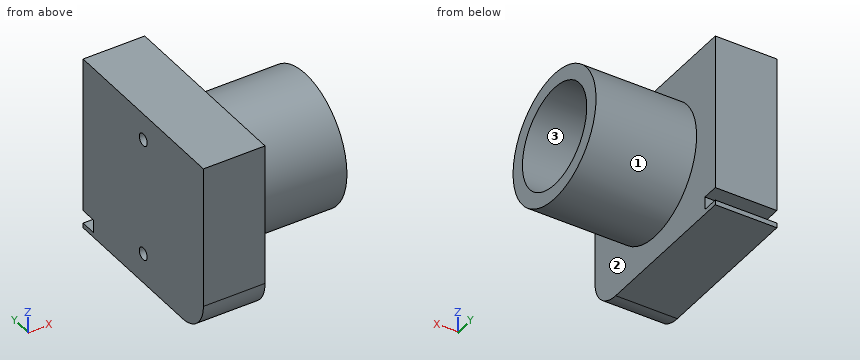
from build123d import *

# Parameters (mm, degrees)
SKETCH1_W           = 19
SKETCH1_H           = 58
BOSS_EXTRUDE1_DEPTH = 54
SKETCH2_3_R         = 20
SKETCH2_3_R_2       = 15.5
BOSS_EXTRUDE2_DEPTH = 50
SKETCH2_R           = 1.9
CUT_EXTRUDE1_DEPTH  = 10
FILLET1_R           = 10
BOSS_EXTRUDE3_DEPTH = 50
SKETCH4_R           = 1.25
CUT_EXTRUDE2_DEPTH  = 55
SKETCH5_W           = 17
SKETCH5_H           = 14
CUT_EXTRUDE3_DEPTH  = 2
SKETCH6_W           = 19
SKETCH6_H           = 4
CUT_EXTRUDE4_DEPTH  = 5
SKETCH7_W           = 17
SKETCH7_H           = 14
CUT_EXTRUDE5_DEPTH  = 53


with BuildPart() as part:
    # Sketch1 → Boss-Extrude1 (new body)
    with BuildSketch(Plane.XY):
        with Locations((9.5, 29)):
            Rectangle(SKETCH1_W, SKETCH1_H)
    extrude(amount=BOSS_EXTRUDE1_DEPTH)

    # Sketch2<3> → Boss-Extrude2 (add)
    with BuildSketch(Plane.ZY):
        with Locations((27.5, 29)):
            Circle(SKETCH2_3_R)
        with Locations((27.5, 29)):
            Circle(SKETCH2_3_R_2, mode=Mode.SUBTRACT)
    extrude(amount=-BOSS_EXTRUDE2_DEPTH)

    # Sketch2 → Cut-Extrude1 (cut)
    with BuildSketch(Plane.ZY):
        with Locations((9.25, 29)):
            Circle(SKETCH2_R)
        with Locations((45.75, 29)):
            Circle(SKETCH2_R)
    extrude(amount=-CUT_EXTRUDE1_DEPTH, mode=Mode.SUBTRACT)

    # Fillet1
    fillet1_edges = [part.edges().sort_by_distance(p)[0] for p in [
        (9.5, 0, 0),
    ]]
    fillet(fillet1_edges, radius=FILLET1_R)

    # Sketch3 → Boss-Extrude3 (add)
    with BuildSketch(Plane(origin=(0, 0, 0), x_dir=(0, 0, -1), z_dir=(1, 0, 0))):
        Polygon((0, 0), (0, 57), (0, 67), (-5, 67), (-5, 0), align=None)
    extrude(amount=-BOSS_EXTRUDE3_DEPTH)

    # Sketch4 → Cut-Extrude2 (cut, through all)
    with BuildSketch(Plane(origin=(0, 0, 0), x_dir=(-1, 0, 0), z_dir=(0, 0, -1))):
        with Locations((14, 57)):
            Circle(SKETCH4_R)
        Polygon((0, 53), (0, 0), (50, 0), (50, 67), (17, 67), (17, 53), align=None)
        with Locations((14, 63.5)):
            Circle(SKETCH4_R)
    extrude(amount=-CUT_EXTRUDE2_DEPTH, mode=Mode.SUBTRACT)

    # Sketch5 → Cut-Extrude3 (cut)
    with BuildSketch(Plane(origin=(0, 0, 0), x_dir=(-1, 0, 0), z_dir=(0, 0, -1))):
        with Locations((8.5, 60)):
            Rectangle(SKETCH5_W, SKETCH5_H)
    extrude(amount=-CUT_EXTRUDE3_DEPTH, mode=Mode.SUBTRACT)

    # Sketch6 → Cut-Extrude4 (cut)
    with BuildSketch(Plane(origin=(0, 58, 0), x_dir=(1, 0, 0), z_dir=(0, 1, 0))):
        with Locations((9.5, -3.5)):
            Rectangle(SKETCH6_W, SKETCH6_H)
    extrude(amount=-CUT_EXTRUDE4_DEPTH, mode=Mode.SUBTRACT)

    # Sketch7 → Cut-Extrude5 (cut, through all)
    with BuildSketch(Plane(origin=(0, 0, 2), x_dir=(-1, 0, 0), z_dir=(0, 0, -1))):
        with Locations((8.5, 60)):
            Rectangle(SKETCH7_W, SKETCH7_H)
    extrude(amount=-CUT_EXTRUDE5_DEPTH, mode=Mode.SUBTRACT)


solid = part.part
Check sheet for the modelled part. Datum: model origin and axes. Units: mm. Face numbers are marked on the shaded views. Give positions to 0.01 mm unless a question says otherwise; leave off trailing zeros. Write each loop counter-clockwise with the first axis right and the second up, starting at its lowest first coordinate (ties: lowest second). Pieces come first, ordered by that corner, then holes. Notation, with made-up numbers: (29, -3) -> (47, -3) arc R33 cw to (47, 25) -> close; hole circle Ø1 at (89.25, 85.25). An arc over 180 degrees is marked (long way). Use one line per item in the form item = value. Start each with the question number.
1. Mould release check, pull along Y, two halves, no side actions. Record for the marked faces 1, 2 and 3: pulls with the +Y half, pulls with the -Y half, needs draft (parallel to the pull), parting line crosses it, or undercut.
2. Section check D-D (z = 24). Record the cut outline in (x, y).
3. Section check A-A (y = 29). Record the cut outline in (x, z).
4. Section check C-C (x = 47). Record the cut outline in (y, z), and give its area (3 significant figures).
5. Go/stop test with flat-tipped pins: P1, Ø1.5, axis at x = 23.5, z = 38.5, coming from the -Y side; P2, Ø12, axis at y = 29, z = 36.5, coming from the +X side; P3, Ø1.9, axis at y = 29.5, z = 46, coming from the -X side; P4, Ø4, axis at y = 50.5, z = 38.5, coming from the -X side. Record where each tip stops, or that it passes through.
6. Thickness scan on line 1 along Y through (x, z) = (26.5, 28); line 2 along Z through (x, y) = (42.5, 43); line 3 along X through (y, z) = (31.5, 25.5). Record the ranges inside material, lowest first. Write a range as from..to.
7. Section check B-B (z = 34). Record the cut outline in (x, y), and give its area (3 significant figures).
Conclusion:
q1.face_1 = parting line crosses it
q1.face_2 = needs draft
q1.face_3 = undercut
q2.outline = (0, 0) -> (19, 0) -> (19, 9.31) -> (50, 9.31) -> (50, 13.9) -> (19, 13.9) -> (19, 44.1) -> (50, 44.1) -> (50, 48.69) -> (19, 48.69) -> (19, 58) -> (0, 58) -> close
q3.outline = (0, 0) -> (19, 0) -> (19, 7.5) -> (50, 7.5) -> (50, 12) -> (19, 12) -> (19, 43) -> (50, 43) -> (50, 47.5) -> (19, 47.5) -> (19, 54) -> (0, 54) -> (0, 47.65) -> (10, 47.65) -> (10, 43.85) -> (0, 43.85) -> (0, 11.15) -> (10, 11.15) -> (10, 7.35) -> (0, 7.35) -> close
q4.outline = circle Ø40 at (29, 27.5); hole circle Ø31 at (29, 27.5)
q4.area = 502 mm²
q5.P1 = 11.83
q5.P2 = 19
q5.P3 = 10
q5.P4 = 0
q6.line_1 = 9.01..13.51, 44.49..48.99
q6.line_2 = 13.22..20.85, 34.15..41.78
q6.line_3 = 0..19
q7.outline = (0, 0) -> (19, 0) -> (19, 10.09) -> (50, 10.09) -> (50, 14.93) -> (19, 14.93) -> (19, 43.07) -> (50, 43.07) -> (50, 47.91) -> (19, 47.91) -> (19, 58) -> (0, 58) -> close
q7.area = 1,400 mm²
